```python
from build123d import *

# Parameters (mm, degrees)
CYLINDER001_R     = 2
CYLINDER001_DEPTH = 10
CYLINDER_R        = 2
CYLINDER_DEPTH    = 10
BOX003_W          = 2
BOX003_H          = 30
BOX003_DEPTH      = 20
FILLET004_R       = 3
CYLINDER003_R     = 2
CYLINDER003_DEPTH = 10
CYLINDER002_R     = 2
CYLINDER002_DEPTH = 10
BOX004_W          = 2
BOX004_H          = 30
BOX004_DEPTH      = 20
FILLET005_R       = 3
BOX002_W          = 30
BOX002_H          = 40
BOX002_DEPTH      = 10
FILLET001_R       = 3
BOX001_W          = 30
BOX001_H          = 20
BOX001_DEPTH      = 10
FILLET_R          = 3
BOX_W             = 50
BOX_H             = 100
BOX_DEPTH         = 2
FILLET002_R       = 3
FILLET003_R       = 3
FILLET006_R       = 2
FILLET007_R       = 2


with BuildPart() as cilindre001:
    # Cylinder001 → Cylinder001 (new body)
    with BuildSketch(Plane(origin=(-10, 23, 13), x_dir=(0, 0, 1), z_dir=(-1, 0, 0))):
        Circle(CYLINDER001_R)
    extrude(amount=CYLINDER001_DEPTH)


with BuildPart() as cilindre:
    # Cylinder → Cylinder (new body)
    with BuildSketch(Plane(origin=(-10, 5, 13), x_dir=(0, 0, 1), z_dir=(-1, 0, 0))):
        Circle(CYLINDER_R)
    extrude(amount=CYLINDER_DEPTH)


with BuildPart() as cut003:
    # Box003 → Box003 (new body)
    with BuildSketch(Plane(origin=(-14, 0, 0), x_dir=(1, 0, 0), z_dir=(0, 0, 1))):
        with Locations((1, 15)):
            Rectangle(BOX003_W, BOX003_H)
    extrude(amount=BOX003_DEPTH)

    # Fillet004
    fillet004_edges = [cut003.edges().sort_by_distance(p)[0] for p in [
        (-13, 0, 20),
        (-13, 30, 20),
    ]]
    fillet(fillet004_edges, radius=FILLET004_R)

    # Cut002: cut Cilindre
    add(cilindre.part, mode=Mode.SUBTRACT)

    # Cut003: cut Cilindre001
    add(cilindre001.part, mode=Mode.SUBTRACT)


with BuildPart() as cut003_1:
    # Cut003 placement: moved
    add(cut003.part.moved(Location((12, 0, 0))))


with BuildPart() as cilindre003:
    # Cylinder003 → Cylinder003 (new body)
    with BuildSketch(Plane(origin=(-10, 23, 13), x_dir=(0, 0, 1), z_dir=(-1, 0, 0))):
        Circle(CYLINDER003_R)
    extrude(amount=CYLINDER003_DEPTH)


with BuildPart() as cilindre002:
    # Cylinder002 → Cylinder002 (new body)
    with BuildSketch(Plane(origin=(-10, 5, 13), x_dir=(0, 0, 1), z_dir=(-1, 0, 0))):
        Circle(CYLINDER002_R)
    extrude(amount=CYLINDER002_DEPTH)


with BuildPart() as cut005:
    # Box004 → Box004 (new body)
    with BuildSketch(Plane(origin=(-14, 0, 0), x_dir=(1, 0, 0), z_dir=(0, 0, 1))):
        with Locations((1, 15)):
            Rectangle(BOX004_W, BOX004_H)
    extrude(amount=BOX004_DEPTH)

    # Fillet005
    fillet005_edges = [cut005.edges().sort_by_distance(p)[0] for p in [
        (-13, 0, 20),
        (-13, 30, 20),
    ]]
    fillet(fillet005_edges, radius=FILLET005_R)

    # Cut004: cut Cilindre002
    add(cilindre002.part, mode=Mode.SUBTRACT)

    # Cut005: cut Cilindre003
    add(cilindre003.part, mode=Mode.SUBTRACT)


with BuildPart() as cut005_1:
    # Cut005 placement: moved
    add(cut005.part.moved(Location((64, 0, 0))))


with BuildPart() as fillet001:
    # Box002 → Box002 (new body)
    with BuildSketch(Plane(origin=(10, 10, -2), x_dir=(1, 0, 0), z_dir=(0, 0, 1))):
        with Locations((15, 20)):
            Rectangle(BOX002_W, BOX002_H)
    extrude(amount=BOX002_DEPTH)

    # Fillet001
    fillet001_edges = [fillet001.edges().sort_by_distance(p)[0] for p in [
        (10, 10, 3),
        (10, 50, 3),
        (40, 10, 3),
        (40, 50, 3),
    ]]
    fillet(fillet001_edges, radius=FILLET001_R)


with BuildPart() as fillet_body:
    # Box001 → Box001 (new body)
    with BuildSketch(Plane(origin=(10, 70, 0), x_dir=(1, 0, 0), z_dir=(0, 0, 1))):
        with Locations((15, 10)):
            Rectangle(BOX001_W, BOX001_H)
    extrude(amount=BOX001_DEPTH)

    # Fillet
    fillet_edges = [fillet_body.edges().sort_by_distance(p)[0] for p in [
        (10, 70, 5),
        (10, 90, 5),
        (40, 70, 5),
        (40, 90, 5),
    ]]
    fillet(fillet_edges, radius=FILLET_R)


with BuildPart() as fillet_body_1:
    # Fillet placement: moved
    add(fillet_body.part.moved(Location((0, 0, -5))))


with BuildPart() as fillet007:
    # Box → Box (new body)
    with BuildSketch(Plane.XY):
        with Locations((25, 50)):
            Rectangle(BOX_W, BOX_H)
    extrude(amount=BOX_DEPTH)

    # Cut: cut Fillet body
    add(fillet_body_1.part, mode=Mode.SUBTRACT)

    # Cut001: cut Fillet001
    add(fillet001.part, mode=Mode.SUBTRACT)

    # Fillet002
    fillet002_edges = [fillet007.edges().sort_by_distance(p)[0] for p in [
        (50, 100, 1),
    ]]
    fillet(fillet002_edges, radius=FILLET002_R)

    # Fillet003
    fillet003_edges = [fillet007.edges().sort_by_distance(p)[0] for p in [
        (0, 100, 1),
    ]]
    fillet(fillet003_edges, radius=FILLET003_R)

    # Fusion: union Cut003, Cut005
    add(cut003_1.part)
    add(cut005_1.part)

    # Fillet006
    fillet006_edges = [fillet007.edges().sort_by_distance(p)[0] for p in [
        (-2, 15, 0),
    ]]
    fillet(fillet006_edges, radius=FILLET006_R)

    # Fillet007
    fillet007_edges = [fillet007.edges().sort_by_distance(p)[0] for p in [
        (52, 15, 0),
    ]]
    fillet(fillet007_edges, radius=FILLET007_R)


solid = fillet007.part
```
For this review, take the finished solid that the model builds, in its own axes (mm). A direction names the side the tool comes from. Round coordinates to 2 decimals unless told otherwise and drop trailing zeros. Write each loop counter-clockwise with the first axis right and the second up, starting at its lowest first coordinate (ties: lowest second). Pieces come first, ordered by that corner, then holes. Notation, with made-up numbers: (-34, 41.5) -> (-28, 41.5) arc R19 ccw to (-28, 48.5) -> close; hole circle Ø7 at (53.25, 54.25). An arc over 180 degrees is marked (long way). One line per question, with ' | ' between items. Start each with the question number.
1) Wall thickness on line 1 along Y through (x, z) = (-1.55, 13); line 2 along X through (y, z) = (22, 5); line 3 along Z through (x, y) = (49, 15.5): over which ranges is each line inside the solid? List them lowest first.
2) Add section A-A (y = 85.5). Write out the cut boundary in (x, z).
3) Machinability: for faces 4 (the cylindrical face through (51.01, 0.86, 19.1)), 5 (the cylindrical face through (39.1, 10.86, 1.01)), which of the approach directions +Z, -Z, +X, -X, +Y, -Y give a long, thin tool a straight path to every point of the face, cutting with its end or side? Answer none if there is none.
4) Mouldability with a two-part tool opening along Z and no side actions: class faces 1 (the cylindrical face through (-1, 5, 11)), 2 (the flat face through (25, 50, 1)), 3 (the flat face through (51, 15, 20)) as +Z half, -Z half, draft (parallel to the pull), parting line (faces both ways), or undercut.
5) Add section D-D (x = 35). Write out the cut boundary in (y, z).
6) For pin 1 Ø1 at (x, z) = (51, 7) entering from +Y; pin 2 Ø1.6 at (y, z) = (23.5, 0.5) entering from -X; pin 3 Ø2 at (y, z) = (78, 1.5) entering from +X; pin 4 Ø8 at (y, z) = (38.5, 7.5) entering from -X, all flat-tipped, find the tip position at first contact; note any pin that passes through.
7) Add section C-C (y = 5). Write out the cut boundary in (x, z).
8) Add section B-B (z = 8). Write out the cut boundary in (x, y).
Reported:
1) line 1: y = 0 to 3, 7 to 21, 25 to 30 | line 2: x = -2 to 0, 50 to 52 | line 3: z = 0 to 2
2) outline: (0, 0) -> (10, 0) -> (10, 2) -> (0, 2) -> close; (40, 0) -> (50, 0) -> (50, 2) -> (40, 2) -> close
3) face 4: +Z, +X, -X, -Y | face 5: +Z, -Z
4) face 1: undercut | face 2: draft | face 3: +Z half
5) outline: (0, 0) -> (10, 0) -> (10, 2) -> (0, 2) -> close; (50, 0) -> (70, 0) -> (70, 2) -> (50, 2) -> close; (90, 0) -> (100, 0) -> (100, 2) -> (90, 2) -> close
6) pin 1: stops at y = 30 | pin 2: stops at x = -1.87 | pin 3: stops at x = 50 | pin 4: passes through
7) outline: (-2, 2) arc R2 ccw to (0, 0) -> (50, 0) arc R2 ccw to (52, 2) -> (52, 11) -> (50, 11) -> (50, 2) -> (0, 2) -> (0, 11) -> (-2, 11) -> close; (-2, 15) -> (0, 15) -> (0, 20) -> (-2, 20) -> close; (50, 15) -> (52, 15) -> (52, 20) -> (50, 20) -> close
8) outline: (-2, 0) -> (0, 0) -> (0, 30) -> (-2, 30) -> close; (50, 0) -> (52, 0) -> (52, 30) -> (50, 30) -> close
